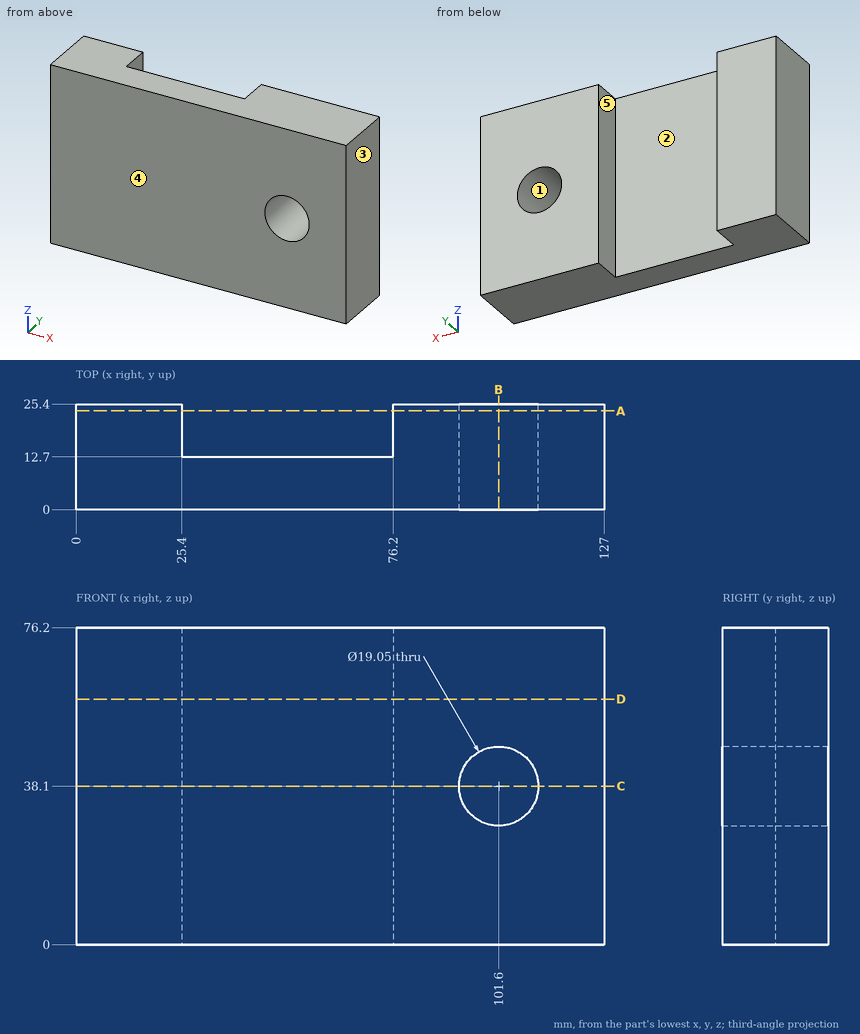
For this review, use the dimensioned drawing (mm, ordinates from the lowest corner) and the shaded views. A direction names the side the tool comes from. Round coordinates to 2 decimals unless told otherwise and drop trailing zeros. Write each loop counter-clockwise with the first axis right and the second up, starting at its lowest first coordinate (ties: lowest second). Pieces come first, ordered by that corner, then holes. Notation, with made-up numbers: M 23.5,-32 L 64.5,-32 A18 ccw 64.5,-2 Z; hole C -32,-23 d6. An arc over 180 degrees is marked long. Write item = value, one per line. Start each with the question number.
(1) We need section B-B (x = 101.6). Give the boundary of the cut face in (y, z) (3 decimals).
(2) We need section D-D (z = 59). Give the boundary of the cut face in (x, y), then the cut area to 3 significant figures.
(3) The part is to be moulded in two halves that separate along X. For the marked faces 3, 4 and 5, say which applies: +X half, -X half, draft (parallel to the pull), parting line (faces both ways), or undercut.
(4) We need section C-C (z = 38.1). Give the boundary of the cut face in (x, y) (3 decimals), then the cut area to 3 significant figures.
(5) For line 1 along X through (y, z) = (19.25, 38.1) (3 decimals); line 2 along X through (y, z) = (14.5, 44); line 3 along X through (y, z) = (7.5, 38.1) (3 decimals), list the stretches that pass through material, from the lowest coordinate up.
(6) We need section A-A (y = 23.75). Give the boundary of the cut face in (x, z) (3 decimals), then the cut area to 3 significant figures.
(7) For the marked faces 1 and 2, list the 3-axis set-ups (+Z, -Z, +X, -X, +Y, -Y) from which the entire face can be reached by the end or side of a thin tool; tool diameter is ignored.
Results found:
q1.outline = M 0,0 L 25.4,0 L 25.4,28.575 L 0,28.575 Z; M 0,47.625 L 25.4,47.625 L 25.4,76.2 L 0,76.2 Z
q2.outline = M 0,0 L 127,0 L 127,25.4 L 76.2,25.4 L 76.2,12.7 L 25.4,12.7 L 25.4,25.4 L 0,25.4 Z
q2.area = 2,580 mm²
q3.face_3 = +X half
q3.face_4 = draft
q3.face_5 = undercut
q4.outline = M 0,0 L 92.075,0 L 92.075,25.4 L 76.2,25.4 L 76.2,12.7 L 25.4,12.7 L 25.4,25.4 L 0,25.4 Z; M 111.125,0 L 127,0 L 127,25.4 L 111.125,25.4 Z
q4.area = 2,100 mm²
q5.line_1 = 0 to 25.4, 76.2 to 92.075, 111.125 to 127
q5.line_2 = 0 to 25.4, 76.2 to 94.12, 109.08 to 127
q5.line_3 = 0 to 92.075, 111.125 to 127
q6.outline = M 0,0 L 25.4,0 L 25.4,76.2 L 0,76.2 Z; M 76.2,0 L 127,0 L 127,76.2 L 76.2,76.2 Z; hole C 101.6,38.1 d19.05
q6.area = 5,520 mm²
q7.face_1 = +Y, -Y
q7.face_2 = +Z, -Z, +Y
